Geometry: final body of the model. Coordinates: model frame, mm. Give positions to 0.01 mm unless a question says otherwise; leave off trailing zeros. Loops run counter-clockwise (first coordinate to the right, second up) from the corner with the lowest first, then second, coordinate; pieces in that order, holes last. Notation, with made-up numbers: (47, 84.5) -> (86, 84.5) arc R22 cw to (86, 107.5) -> close; hole circle Ø2 at (52.5, 87). An arc over 180 degrees is marked (long way). Answer in a Markdown table with one row per item. Add a question column.
1) Section query D-D (x = 112.5). Return the cut outline in (y, z).
2) Line query: line 1 (Y direction, x = 155, z = -0.05); line 2 (X direction, y = 87.5, z = 0.4); line 3 (X direction, y = 82, z = 0.95). Output: solid intervals per line, ascending. Write a range as from..to.
3) Section query C-C (y = 33). Return the cut outline in (x, z).
4) Section query A-A (z = -0.2). Give the number of separate pieces and of enclosed holes in the cut face, plus the area to 3 significant figures.
5) Section query B-B (y = 64). Return the cut outline in (x, z), plus the area to 3 significant figures.
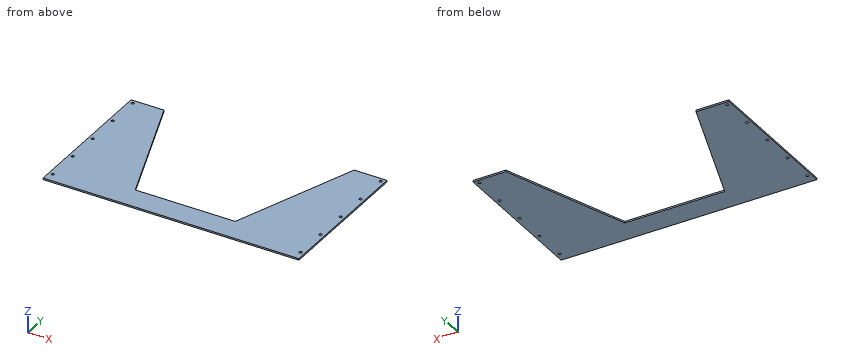
```python
from build123d import *

# Parameters (mm, degrees)
EXTRUDE_1_DEPTH     = 1
SKETCH_2_R          = 1.7
CUT_EXTRUDE_1_DEPTH = 10


with BuildPart() as part:
    # Эскиз1 → Бобышка-Вытянуть1 (new, symmetric)
    with BuildSketch(Plane.XY):
        Polygon((-118.915386311, 92.5), (-62.5, -62.5), (62.5, -62.5), (118.915386311, 92.5), (160, 92.5), (160, -92.5), (-160, -92.5), (-160, 92.5), align=None)
    extrude(amount=EXTRUDE_1_DEPTH, both=True)

    # Эскиз2 → Вырез-Вытянуть1 (cut)
    with BuildSketch(Plane.XY.offset(1)):
        with Locations((-155, 87.5)):
            Circle(SKETCH_2_R)
        with Locations((-155, 45.5)):
            Circle(SKETCH_2_R)
        with Locations((-155, 3.5)):
            Circle(SKETCH_2_R)
        with Locations((-155, -38.5)):
            Circle(SKETCH_2_R)
        with Locations((-155, -80.5)):
            Circle(SKETCH_2_R)
        with Locations((155, -80.5)):
            Circle(SKETCH_2_R)
        with Locations((155, -38.5)):
            Circle(SKETCH_2_R)
        with Locations((155, 3.5)):
            Circle(SKETCH_2_R)
        with Locations((155, 45.5)):
            Circle(SKETCH_2_R)
        with Locations((155, 87.5)):
            Circle(SKETCH_2_R)
    extrude(amount=-CUT_EXTRUDE_1_DEPTH, mode=Mode.SUBTRACT)


solid = part.part
```
Evaluation:
| question | item | result |
|---|---|---|
| 1 | outline | (-92.5, -1) -> (74.87, -1) -> (74.87, 1) -> (-92.5, 1) -> close |
| 2 | line 1 | -92.5..-82.2, -78.8..-40.2, -36.8..1.8, 5.2..43.8, 47.2..85.8, 89.2..92.5 |
| 2 | line 2 | -160..-156.7, -153.3..-117.1, 117.1..153.3, 156.7..160 |
| 2 | line 3 | -160..-115.09, 115.09..160 |
| 3 | outline | (-160, -1) -> (-97.26, -1) -> (-97.26, 1) -> (-160, 1) -> close; (97.26, -1) -> (160, -1) -> (160, 1) -> (97.26, 1) -> close |
| 4 | separate pieces | 1 |
| 4 | enclosed holes | 10 |
| 4 | area | 31,000 mm² |
| 5 | outline | (-160, -1) -> (-108.54, -1) -> (-108.54, 1) -> (-160, 1) -> close; (108.54, -1) -> (160, -1) -> (160, 1) -> (108.54, 1) -> close |
| 5 | area | 206 mm² |
